Could you check a few things on this model? Use its own coordinates, in mm. Coordinates: 2 decimals unless noted, no trailing zeros. Order: outer loops, then holes, each group sorted by start corner. A loop starts at its lowest first (then second) coordinate and runs counter-clockwise, first axis right, second up. Notation, with made-up numbers: (14, 53) -> (21, 53) arc R27 ccw to (21, 86) -> close; hole circle Ø4 at (70, 58.25). An arc over 180 degrees is marked (long way). Put each result on its own line as item: value. Start each with the question number.
Q1. If we section it at C-C (y = 15.5): Please give me the cut outline in (x, z).
Q2. Please list where these lines run through material, in increasing order: line 1 along Z through (x, y) = (0, 19.75); line 2 along X through (y, z) = (7.25, -13.5); line 3 along Z through (x, y) = (-10, 21.5).
Q3. If we section it at A-A (x = 0): Please give me the cut outline in (y, z), and give its area (3 significant figures).
Q4. We'd pull the mould along X, two halves only. Please class faces 1 (the face through (-1, 12, -40)), 2 (the face through (-40, 12, 1)), 3 (the face through (-28, 12, -21)): +X half, -X half, draft (parallel to the pull), parting line (faces both ways), or undercut.
Q5. If we section it at B-B (z = 0): Please give me the cut outline in (x, y).
from build123d import *

# Parameters (mm, degrees)
SKETCH1_W           = 80
SKETCH1_H           = 80
BOSS_EXTRUDE1_DEPTH = 25
SKETCH2_R           = 35
CUT_EXTRUDE1_DEPTH  = 26


with BuildPart() as part:
    # Sketch1 → Boss-Extrude1 (new body)
    with BuildSketch(Plane(origin=(0, 0, 0), x_dir=(1, 0, 0), z_dir=(0, 1, 0))):
        Rectangle(SKETCH1_W, SKETCH1_H)
    extrude(amount=BOSS_EXTRUDE1_DEPTH)

    # Sketch2 → Cut-Extrude1 (cut, through all)
    with BuildSketch(Plane.XZ):
        Circle(SKETCH2_R)
    extrude(amount=-CUT_EXTRUDE1_DEPTH, mode=Mode.SUBTRACT)


solid = part.part
The answers:
1. outline: (-40, -40) -> (40, -40) -> (40, 40) -> (-40, 40) -> close; hole circle Ø70 at (0, 0)
2. line 1: -40 to -35, 35 to 40
2. line 2: -40 to -32.29, 32.29 to 40
2. line 3: -40 to -33.54, 33.54 to 40
3. outline: (0, -40) -> (25, -40) -> (25, -35) -> (0, -35) -> close; (0, 35) -> (25, 35) -> (25, 40) -> (0, 40) -> close
3. area: 250 mm^2
4. face 1: draft
4. face 2: -X half
4. face 3: undercut
5. outline: (-40, 0) -> (-35, 0) -> (-35, 25) -> (-40, 25) -> close; (35, 0) -> (40, 0) -> (40, 25) -> (35, 25) -> close
